Input: part model. Units: mm. Frame: model coordinates. A direction names the side the tool comes from. Round coordinates to 2 decimals unless told otherwise and drop trailing zeros. Loops run counter-clockwise (first coordinate to the right, second up) from the corner with the lowest first, then second, coordinate; pieces in that order, holes last.
(1) Access query for faces 4 (the face through (-7, 5, 0)), 5 (the face through (12.258, 2, 0)). Directions: +Z, -Z, +X, -X, +Y, -Y. A direction counts if a zero-diameter tool reaches every point of the face in a straight line with its end or side. Return the directions, or none.
(2) Line query: line 1 (X direction, y = 3.8, z = 0); line 2 (X direction, y = 9, z = 0); line 3 (Y direction, x = -16.5, z = -4.25). Output: solid intervals per line, ascending.
(3) Cut plane C-C, the plane y = 7.75. Output: boundary loops of the cut face in (x, z).
(4) First-contact query: pin 1 Ø4 at (x, z) = (7.18, 0) entering from +Y; pin 2 Ø10 at (x, z) = (7, 9) entering from +Y; pin 3 Ø6 at (y, z) = (10.5, 5.5) entering from +X. Flat tips, straight axial feed; report the tip coordinate or a pass-through.
(5) Cut plane B-B, the plane x = -22. Output: boundary loops of the cut face in (y, z).
(6) Draft query along Z for faces 1 (the face through (-4.358, 9.462, 3.174)), 2 (the face through (-7, 2, -12.7)), 3 (the face through (-11, 5, -6)). Return one class per face: released by +Z, released by -Z, zero draft, split by the parting line, or undercut.
(7) Cut plane A-A, the plane z = 0. Output: boundary loops of the cut face in (x, y).
from build123d import *

# Parameters (mm, degrees)
SKETCH1_W           = 38.1
SKETCH1_H           = 25.4
BOSS_EXTRUDE1_DEPTH = 5
SKETCH3_R           = 7
SKETCH3_R_2         = 4
BOSS_EXTRUDE2_DEPTH = 9.05
SKETCH4_R           = 3.5
CUT_EXTRUDE1_DEPTH  = 31.182577446


with BuildPart() as part:
    # Sketch1 → Boss-Extrude1 (new body)
    with BuildSketch(Plane(origin=(0, 0, 0), x_dir=(1, 0, 0), z_dir=(0, 1, 0))):
        with Locations((-6.79173913, 0)):
            Rectangle(SKETCH1_W, SKETCH1_H)
    extrude(amount=BOSS_EXTRUDE1_DEPTH)

    # Sketch3 → Boss-Extrude2 (add)
    with BuildSketch(Plane(origin=(0, 5, 0), x_dir=(1, 0, 0), z_dir=(0, 1, 0))):
        with Locations(Location((-6.79173913, 0, 0), (0, 0, 90))):
            Circle(SKETCH3_R)
        with Locations(Location((-6.79173913, 0, 0), (0, 0, 90))):
            Circle(SKETCH3_R_2, mode=Mode.SUBTRACT)
    extrude(amount=BOSS_EXTRUDE2_DEPTH)

    # Sketch4 → Cut-Extrude1 (cut, through all)
    with BuildSketch(Plane(origin=(0, 5, 0), x_dir=(1, 0, 0), z_dir=(0, 1, 0))):
        with Locations(Location((7.17826087, 0, 0), (0, 0, 270))):
            Circle(SKETCH4_R)
        with Locations(Location((-20.76173913, 0, 0), (0, 0, 270))):
            Circle(SKETCH4_R)
    extrude(amount=-CUT_EXTRUDE1_DEPTH, mode=Mode.SUBTRACT)


solid = part.part
Reported:
1. face 4: +Y
1. face 5: +Z, -Z, +X, +Y, -Y
2. line 1: x = -25.84 to -24.26, -17.26 to 3.68, 10.68 to 12.26
2. line 2: x = -13.79 to -10.79, -2.79 to 0.21
2. line 3: y = 0 to 5
3. outline: circle Ø14 at (-6.79, 0); hole circle Ø8 at (-6.79, 0)
4. pin 1: passes through
4. pin 2: stops at y = 5
4. pin 3: stops at x = -0.25
5. outline: (0, -12.7) - (5, -12.7) - (5, -3.27) - (0, -3.27) - close; (0, 3.27) - (5, 3.27) - (5, 12.7) - (0, 12.7) - close
6. face 1: undercut
6. face 2: released by -Z
6. face 3: zero draft
7. outline: (-25.84, 0) - (-24.26, 0) - (-24.26, 5) - (-25.84, 5) - close; (-17.26, 0) - (3.68, 0) - (3.68, 5) - (0.21, 5) - (0.21, 14.05) - (-2.79, 14.05) - (-2.79, 5) - (-10.79, 5) - (-10.79, 14.05) - (-13.79, 14.05) - (-13.79, 5) - (-17.26, 5) - close; (10.68, 0) - (12.26, 0) - (12.26, 5) - (10.68, 5) - close
